Verification items for the finished model (mm, model axes). A direction names the side the tool comes from. Round coordinates to 2 decimals unless told otherwise and drop trailing zeros. Loops run counter-clockwise (first coordinate to the right, second up) from the corner with the lowest first, then second, coordinate; pieces in that order, holes last. Notation, with made-up numbers: M 14,64.25 L 40,64.25 A4 ccw 40,70.25 Z; hole C 46,-27 d9. An arc over 180 degrees is marked long. Answer as CSV lines item,"result".
Autodesk Inventor part; units mm, degrees
ref_plane "YZ Plane" through (0, 0, 0) normal (1, 0, 0) x (0, 1, 0)
ref_plane "XZ Plane" through (0, 0, 0) normal (0, 1, 0) x (-1, 0, 0)
ref_plane "XY Plane" through (0, 0, 0) normal (0, 0, 1) x (1, 0, 0)
sketch "草圖1" plane through (0, 0, 0) normal (0, 1, 0) x (-1, 0, 0)
  line L0 (0, 0) -> (-70, 0)
  line L1 (-70, 0) -> (-70, -40)
  line L2 (-70, -40) -> (0, -40)
  line L3 (0, -40) -> (0, 0)
  dimension "d0" = 40
  dimension "d1" = 70
extrude "擠出1" add sketch "草圖1" along normal blind 20
sketch "草圖2" plane through (0, 20, 0) normal (0, 1, 0) x (1, 0, 0)
  line L0 (0, 0) -> (70, 0)
  line L1 (20, 0) -> (30, 0)
  line L2 (30, 0) -> (30, 10)
  line L3 (30, 10) -> (20, 10)
  line L4 (20, 10) -> (20, 0)
  line L5 (70, 40) -> (0, 40)
  line L6 (20, 40) -> (30, 40)
  line L7 (30, 40) -> (30, 30)
  line L8 (30, 30) -> (20, 30)
  line L9 (20, 30) -> (20, 40)
  line L10 (0, 40) -> (0, 0)
  dimension "d4" = 10
  dimension "d5" = 10
  dimension "d6" = 10
  dimension "d7" = 20
extrude "擠出2" cut sketch "草圖2" against normal blind 20
fillet "圓角1" radius 20 2 edges at (70, 10, 0) (70, 10, -40)
hole "孔1" at (50, 20, -20) direction (0, -1, 0) diameter 20 depth 20 tip angle 118
properties part number "32"
1) Go/stop test with flat-tipped pins: pin 1 (5 mm diameter, centred on x = 24, y = 6, fed in from -Z); pin 2 (5 mm diameter, centred on y = 16.5, z = -13, fed in from +X); pin 3 (3 mm diameter, centred on y = 14.5, z = -34.5, fed in from +X). Record where each tip stops, or that it passes through.
Here are the results:
pin 1,"stops at z = -30"
pin 2,"stops at x = 69.49"
pin 3,"stops at x = 65.2"
2) Draft check along X on faces 1 (the cylindrical face through (63.986, 10.14, -5.703)), 2 (the flat face through (0, 10, -20)), 3 (the flat face through (10, 10, 0)), 4 (the flat face through (25, 10, -30)). Enter one of: +X half, -X half, draft (parallel to the pull), parting line (faces both ways), or undercut.
Here are the results:
face 1,"+X half"
face 2,"-X half"
face 3,"draft"
face 4,"undercut"
3) Section check B-B (z = -26). Record the cut outline in (x, y).
Here are the results:
outline,"M 0,0 L 42,0 L 42,20 L 0,20 Z; M 58,0 L 69.08,0 L 69.08,20 L 58,20 Z"
4) Material ranges on probe 1 along Z at (x, y) = (50, 4.75); probe 2 along X at (y, z) = (12.75, -20); probe 3 along X at (y, z) = (4, -36), recorded low to high.
Here are the results:
probe 1,"z = -40 to -30, -10 to 0"
probe 2,"x = 0 to 40, 60 to 70"
probe 3,"x = 0 to 20, 30 to 62"
5) Set-up check for faces 5 (the flat face through (25, 10, -10)), 6 (the flat face through (10, 10, -40)), 7 (the flat face through (30, 10, -35)): record each of +Z, -Z, +X, -X, +Y, -Y from which the full face is reachable in a straight line by a thin tool's end or side.
Here are the results:
face 5,"+Z, +Y, -Y"
face 6,"-Z, +X, -X, +Y, -Y"
face 7,"-Z, +Y, -Y"
6) Section check D-D (x = 62). Record the cut outline in (y, z).
Here are the results:
outline,"M 0,-36 L 20,-36 L 20,-4 L 0,-4 Z"
7) Section check C-C (x = 43.5). Record the cut outline in (y, z).
Here are the results:
outline,"M 0,-40 L 20,-40 L 20,-27.6 L 0,-27.6 Z; M 0,-12.4 L 20,-12.4 L 20,0 L 0,0 Z"
